Build history of the part. All positions in model axes, mm. A direction names the side the tool comes from. Coordinates: 2 decimals unless noted, no trailing zeros. Loops run counter-clockwise (first coordinate to the right, second up) from the corner with the lowest first, then second, coordinate; pieces in that order, holes last. Notation, with made-up numbers: M -3,53.5 L 24,53.5 A14 cw 24,72.5 Z; hole C -24,-39 d1. An arc over 180 degrees is marked long. Write each question's results on one line, items separated by ' | '. Start each with the question number.
from build123d import *

# Parameters (mm, degrees)
F1_R     = 7.366
F2_DEPTH = 9.652
F3_R     = 8.255
F4_DEPTH = 1.778
F5_R     = 7.747
F6_DEPTH = 1.016
F0_R     = 7.112
F7_DEPTH = 19.304


with BuildPart() as f2:
    # F1 (on Top) → F2 (new body)
    with BuildSketch(Plane.XY):
        Circle(F1_R)
    extrude(amount=F2_DEPTH)

    # F3 (on face) → F4 (join)
    with BuildSketch(Plane.XY.offset(9.652)):
        Circle(F3_R)
    extrude(amount=F4_DEPTH)

    # F5 (on face) → F6 (cut)
    with BuildSketch(Plane.XY.offset(11.43)):
        Circle(F5_R)
    extrude(amount=-F6_DEPTH, mode=Mode.SUBTRACT)

    # F0 (on Top) → F7 (cut)
    with BuildSketch(Plane.XY):
        Circle(F0_R)
    extrude(amount=F7_DEPTH, mode=Mode.SUBTRACT)


solid = f2.part
1. Mould opens along Y. For faces 3 (the cylindrical face through (-1.542, -6.943, 5.134)), 4 (the cylindrical face through (7.874, 2.48, 10.529)), 5 (the flat face through (-7, 3, 9.652)) say: +Y half, -Y half, draft (parallel to the pull), parting line (faces both ways), or undercut.
2. Band-saw the part on A-A, the plane y = 0. List the corners of the cut face in (x, z) (3 decimals).
3. Which spindle directions (+Z, -Z, +X, -X, +Y, -Y) get a long thin tool onto all of the face, cutting with end or side? Do faces 1 (the cylindrical face through (4.165, 6.532, 10.929)), 2 (the cylindrical face through (3.399, -6.535, 4.758)). Say none if no direction does.
4. Pin check, flat tips, straight feed: pin 1 (4 mm diameter, centred on x = 1, z = 5.5, fed in from -Y); pin 2 (1 mm diameter, centred on x = 3.5, z = 3.5, fed in from +Y); pin 3 (1 mm diameter, centred on x = 6.5, y = 1.5, fed in from +Z). Stop position of each tip, or through.
5. Wall check: line 1 along X through (y, z) = (-0.25, 2.25); line 2 along Y through (x, z) = (0, 3); line 3 along Y through (x, z) = (0, 10.95) (3 decimals). Give the ranges that are in metal, low to high.
6. Band-saw the part on C-C, the plane z = 4.5. List the corners of the cut face in (x, y), plus the area to 3 significant figures.
Checked values:
1) face 3: undercut | face 4: parting line | face 5: draft
2) outline: M -8.255,9.652 L -7.366,9.652 L -7.366,0 L -7.112,0 L -7.112,10.414 L -7.747,10.414 L -7.747,11.43 L -8.255,11.43 Z; M 7.112,0 L 7.366,0 L 7.366,9.652 L 8.255,9.652 L 8.255,11.43 L 7.747,11.43 L 7.747,10.414 L 7.112,10.414 Z
3) face 1: +Z | face 2: -Z
4) pin 1: y = -7.37 | pin 2: y = 6.73 | pin 3: z = 10.41
5) line 1: -7.36 to -7.11, 7.11 to 7.36 | line 2: -7.37 to -7.11, 7.11 to 7.37 | line 3: -8.255 to -7.747, 7.747 to 8.255
6) outline: C 0,0 d14.73; hole C 0,0 d14.22 | area: 11.6 mm²
